Here's how the part is built. I have some questions about the finished solid (model axes, mm). A direction names the side the tool comes from. Round coordinates to 2 decimals unless told otherwise and drop trailing zeros. Order: outer loops, then holes, each group sorted by start corner. A loop starts at its lowest first (then second) coordinate and runs counter-clockwise, first axis right, second up. Notation, with made-up numbers: M 3.25,-25 L 48.25,-25 A34 cw 48.25,10 Z; hole C -11.5,21.25 d1. An arc over 180 degrees is marked long. Use one line per item in the form item = value. Start each with the question number.
```python
from build123d import *

# Parameters (mm, degrees)
F0_R     = 34.925
F1_DEPTH = 63.5
F2_R     = 57.15
F2_R_2   = 34.925
F3_DEPTH = 6.35
F4_R     = 57.15
F4_R_2   = 50.8
F5_DEPTH = 63.5


with BuildPart() as f1:
    # F0 (on Top) → F1 (new body)
    with BuildSketch(Plane.XY):
        Circle(F0_R)
    extrude(amount=F1_DEPTH)

    # F2 (on face) → F3 (join)
    with BuildSketch(Plane.XY.offset(63.5)):
        Circle(F2_R)
        Circle(F2_R_2, mode=Mode.SUBTRACT)
        Circle(F2_R_2)
    extrude(amount=F3_DEPTH)

    # F4 (on face) → F5 (join)
    with BuildSketch(Plane.XY.offset(69.85)):
        Circle(F4_R)
        Circle(F4_R_2, mode=Mode.SUBTRACT)
    extrude(amount=F5_DEPTH)


solid = f1.part
```
1) If we section it at C-C on z = 101: Write out the boundary of the cut face in (x, y), then the cut area to 3 significant figures.
2) On a 3-axis mill with a long thin cutter (end or side, diameter ignored), from which of +Z, -Z, +X, -X, +Y, -Y can I reach the whole of each face in a straight line? I mean faces 4 (the flat face through (-26, -25, 63.5)), 5 (the flat face through (-1, 1, 69.85)), 6 (the flat face through (-38, -34, 133.35)). Say none if no direction works.
3) If we section it at A-A on y = 0: Write out the boundary of the cut face in (x, z) (3 decimals), then the cut area to 3 significant figures.
4) If we section it at B-B on x = -19: Write out the boundary of the cut face in (y, z).
5) If we mould it in two halves opening along Y, with no side actions, what happens to faces 1 (the cylindrical face through (-11.012, -49.592, 101.155)), 2 (the cylindrical face through (-27.715, -21.251, 31.306)), 3 (the flat face through (0, 0, 0))? For each: +Y half, -Y half, draft (parallel to the pull), parting line (faces both ways), or undercut.
6) Will these pins go through, and if not, where does the flat tip stop? pin 1 Ø1.5 at (y, z) = (12.5, 63.5) entering from +X; pin 2 Ø8 at (x, y) = (-44.5, -29.5) entering from -Z; pin 3 Ø3 at (y, z) = (26.5, 113) entering from +X.
7) If we section it at D-D on z = 22: Write out the boundary of the cut face in (x, y) (3 decimals), then the cut area to 3 significant figures.
8) If I drill on line 1 (Y direction, x = 0, z = 92); line 2 (Z direction, x = -12, y = 0); line 3 (X direction, y = -1, z = 100.5), over which ranges is the centre line in solid material (lowest first)?
Completed:
q1.outline = C 0,0 d114.3; hole C 0,0 d101.6
q1.area = 2,150 mm²
q2.face_4 = -Z
q2.face_5 = +Z
q2.face_6 = +Z, +X, -X, +Y, -Y
q3.outline = M -57.15,63.5 L -34.925,63.5 L -34.925,0 L 34.925,0 L 34.925,63.5 L 57.15,63.5 L 57.15,133.35 L 50.8,133.35 L 50.8,69.85 L -50.8,69.85 L -50.8,133.35 L -57.15,133.35 Z
q3.area = 5,970 mm²
q4.outline = M -53.9,63.5 L -29.3,63.5 L -29.3,0 L 29.3,0 L 29.3,63.5 L 53.9,63.5 L 53.9,133.35 L 47.11,133.35 L 47.11,69.85 L -47.11,69.85 L -47.11,133.35 L -53.9,133.35 Z
q5.face_1 = undercut
q5.face_2 = parting line
q5.face_3 = draft
q6.pin_1 = 55.93
q6.pin_2 = 63.5
q6.pin_3 = 51.39
q7.outline = C 0,0 d69.85
q7.area = 3,830 mm²
q8.line_1 = -57.15 to -50.8, 50.8 to 57.15
q8.line_2 = 0 to 69.85
q8.line_3 = -57.14 to -50.79, 50.79 to 57.14
